Geometry check sheet. Reference: drawing and pictorial views, mm from the part's lowest x, y, z. Coordinates: 2 decimals unless noted, no trailing zeros. Write each loop counter-clockwise with the first axis right and the second up, starting at its lowest first coordinate (ties: lowest second). Pieces come first, ordered by that corner, then holes.
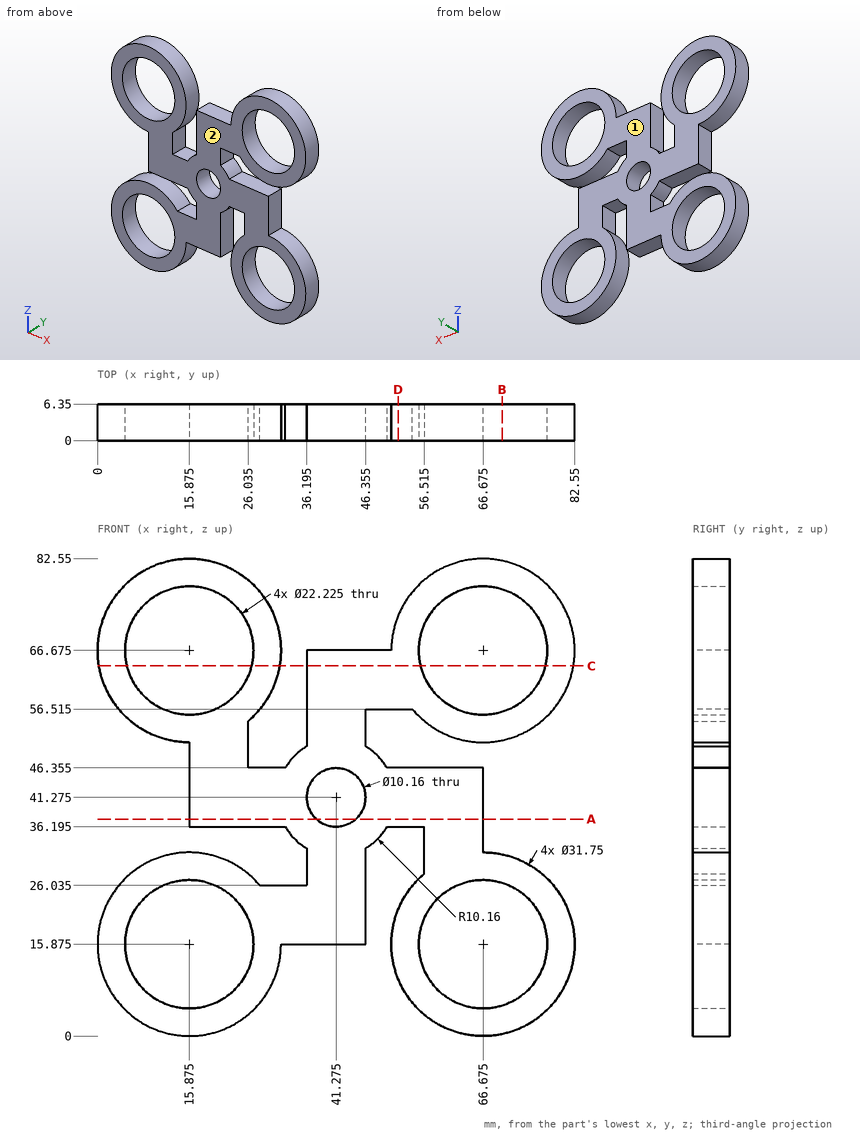
1. Gauge pin test, flat ends, axial feed: P1, Ø1.5, axis at x = 61.5, y = 3.5, coming from the -Z side; P2, Ø1.9, axis at y = 2, z = 28.5, coming from the -X side; P3, Ø3, axis at x = 40, y = 2.5, coming from the -Z side (3 decimals); P4, Ø6, axis at x = 27, z = 28.5, coming from the -Y side. Record the tip position at first contact, or that the pin passes through.
2. Sectioned sample at A-A, the plane z = 37.5. Record the boundary of the cut face in (x, y) (3 decimals), and give its area (3 significant figures).
3. Sectioned sample at B-B, the plane x = 70. Record the boundary of the cut face in (y, z).
4. Sectioned sample at D-D, the plane x = 52. Record the boundary of the cut face in (y, z) (3 decimals).
5. Sectioned sample at C-C, the plane z = 64. Record the boundary of the cut face in (x, y) (3 decimals), and give its area (3 significant figures).
6. Draft check along Y on the marked faces 1 and 2. Enter one of: pulls with the +Y half, pulls with the -Y half, needs draft (parallel to the pull), parting line crosses it, or undercut.
7. Material ranges on L1, parallel to X at y = 1.75, z = 65 (3 decimals); L2, parallel to Z at x = 66.5, y = 1.75 (3 decimals); L3, parallel to Z at x = 19, y = 4.25 (3 decimals), recorded low to high.
Outcome:
1. P1: stops at z = 0.63
1. P2: stops at x = 5.12
1. P3: stops at z = 15.875
1. P4: stops at y = 0
2. outline: (15.875, 0) - (37.876, 0) - (37.876, 6.35) - (15.875, 6.35) - close; (44.674, 0) - (66.675, 0) - (66.675, 6.35) - (44.674, 6.35) - close
2. area: 279 mm2
3. outline: (0, 0.35) - (6.35, 0.35) - (6.35, 5.27) - (0, 5.27) - close; (0, 26.48) - (6.35, 26.48) - (6.35, 31.4) - (0, 31.4) - close; (0, 51.15) - (6.35, 51.15) - (6.35, 56.07) - (0, 56.07) - close; (0, 77.28) - (6.35, 77.28) - (6.35, 82.2) - (0, 82.2) - close
4. outline: (0, 9.82) - (6.35, 9.82) - (6.35, 21.93) - (0, 21.93) - close; (0, 36.195) - (6.35, 36.195) - (6.35, 46.355) - (0, 46.355) - close; (0, 56.515) - (6.35, 56.515) - (6.35, 72.73) - (0, 72.73) - close
5. outline: (0.227, 0) - (5.089, 0) - (5.089, 6.35) - (0.227, 6.35) - close; (26.661, 0) - (31.523, 0) - (31.523, 6.35) - (26.661, 6.35) - close; (36.195, 0) - (55.889, 0) - (55.889, 6.35) - (36.195, 6.35) - close; (77.461, 0) - (82.323, 0) - (82.323, 6.35) - (77.461, 6.35) - close
5. area: 218 mm2
6. face 1: pulls with the +Y half
6. face 2: pulls with the -Y half
7. L1: x = 0.089 to 4.889, 26.861 to 31.661, 36.195 to 55.689, 77.661 to 82.461
7. L2: z = 0.001 to 4.764, 26.986 to 46.355, 50.801 to 55.564, 77.786 to 82.549
7. L3: z = 0.311 to 5.211, 26.539 to 31.439, 36.195 to 56.011, 77.339 to 82.239
